Could you check a few things on this model? Use its own coordinates, in mm. A direction names the side the tool comes from. Coordinates: 2 decimals unless noted, no trailing zeros. Loops run counter-clockwise (first coordinate to the right, second up) from the corner with the lowest first, then second, coordinate; pieces in that order, holes last. Notation, with made-up numbers: (52, 80.5) - (62, 80.5) arc R24 ccw to (62, 94.5) - close; hole circle Ø6 at (28, 30.25). An arc over 180 degrees is marked (long way). One line per question, with ' | ' between items. Start each with the question number.
1. I'm going to push flat-ended pins straight in: P1, Ø4, axis at x = -18, y = 7, coming from the -Z side; P2, Ø1.3, axis at x = 77.5, z = -45, coming from the -Y side; P3, Ø0.6, axis at x = -69.5, y = 4.5, coming from the +Z side; P4, Ø0.5, axis at x = -78, y = 1.5, coming from the +Z side. Where does each tip first touch, or does it pass through?
2. I want a section at C-C, the plane z = 25. Write out the boundary of the cut face in (x, y), then the cut area to 3 significant figures.
3. Which directions (+Z, -Z, +X, -X, +Y, -Y) give clear straight access to the entire face, cutting with the end or side of a thin tool? Please do faces 1 (the flat face through (6, 0, 53)), 2 (the flat face through (-73, 5.4, 16)), 3 (the cylindrical face through (-70.64, -0.25, 50.2)).
4. We'd pull the mould along X, two halves only. Please class faces 4 (the cylindrical face through (-78.35, 4.39, 5.28)), 5 (the flat face through (-0.3, 0.5, -43.2)), 6 (the cylindrical face through (70.6, -0.25, -50.24)): pulls with the +X half, pulls with the -X half, needs draft (parallel to the pull), parting line crosses it, or undercut.
5. I want a section at B-B, the plane x = -55.5. Write out the boundary of the cut face in (y, z).
6. Please list where these lines run through material, in increasing order: L1, parallel to X at y = 0.75, z = -44.85; L2, parallel to X at y = 0.75, z = 29; L3, parallel to X at y = 2.25, z = 37. Write a range as [from, to].
7. I want a section at A-A, the plane z = 13.5. Write out the boundary of the cut face in (x, y), then the cut area to 3 significant figures.
from build123d import *

# Parameters (mm, degrees)
SKETCH1_W                            = 159.7
SKETCH1_H                            = 109.7
BOSS_EXTRUDE1_DEPTH                  = 3.4
SKETCH5_W                            = 128
SKETCH5_H                            = 86
CUT_EXTRUDE1_DEPTH                   = 97.933508138
SKETCH6_W                            = 133.6
SKETCH6_H                            = 96.6
CUT_EXTRUDE2_DEPTH                   = 2.9
F_2_7_2_7_DIAMETER_HOLE1_D           = 2.7
F_2_7_2_7_DIAMETER_HOLE1_CSINK_D     = 2.75
F_2_7_2_7_DIAMETER_HOLE1_CSINK_ANGLE = 90
SKETCH10_R                           = 1.35
BOSS_EXTRUDE3_DEPTH                  = 0.5
M2X0_4_TAPPED_HOLE1_D                = 1.6
M2X0_4_TAPPED_HOLE1_CSINK_D          = 2.05
M2X0_4_TAPPED_HOLE1_CSINK_ANGLE      = 90
SKETCH7_W                            = 143
SKETCH7_H                            = 102.2
SKETCH7_W_2                          = 141
SKETCH7_H_2                          = 100.2
BOSS_EXTRUDE2_DEPTH                  = 0.5
SKETCH17_R                           = 1.5
CUT_EXTRUDE6_DEPTH                   = 2
SKETCH15_W                           = 2.5
SKETCH15_H                           = 4.9
CUT_EXTRUDE5_DEPTH                   = 97.952333649
CUT_EXTRUDE4_DEPTH                   = 97.952333649
SKETCH8_R                            = 8
CUT_EXTRUDE3_DEPTH                   = 97.952333649
SKETCH14_R                           = 2.3
BOSS_EXTRUDE4_DEPTH                  = 7.2
FILLET1_R                            = 8
FILLET2_R                            = 2
FILLET3_R                            = 3
FILLET4_R                            = 1
FILLET5_R                            = 2
FILLET6_R                            = 1
SKETCH16_W                           = 13.05
SKETCH16_H                           = 24
BOSS_EXTRUDE5_DEPTH                  = 2
FILLET7_R                            = 5


with BuildPart() as part:
    # Sketch1 → Boss-Extrude1 (new body)
    with BuildSketch(Plane(origin=(0, 0, 0), x_dir=(1, 0, 0), z_dir=(0, 1, 0))):
        Rectangle(SKETCH1_W, SKETCH1_H)
    extrude(amount=BOSS_EXTRUDE1_DEPTH)

    # Sketch5 → Cut-Extrude1 (cut, through all)
    with BuildSketch(Plane.XZ):
        Rectangle(SKETCH5_W, SKETCH5_H)
    extrude(amount=-CUT_EXTRUDE1_DEPTH, mode=Mode.SUBTRACT)

    # Sketch6 → Cut-Extrude2 (cut)
    with BuildSketch(Plane(origin=(0, 3.4, 0), x_dir=(1, 0, 0), z_dir=(0, 1, 0))):
        Rectangle(SKETCH6_W, SKETCH6_H)
    extrude(amount=-CUT_EXTRUDE2_DEPTH, mode=Mode.SUBTRACT)

    # Ø2.7 (2.7) Diameter Hole1 (through all)
    with Locations(Plane(origin=(0, 3.4, 0), x_dir=(1, 0, 0), z_dir=(0, 1, 0))):
        with Locations((-77.5, 29), (-77.5, -29), (77.5, 29), (77.5, -29)):
            CounterSinkHole(F_2_7_2_7_DIAMETER_HOLE1_D / 2, F_2_7_2_7_DIAMETER_HOLE1_CSINK_D / 2, counter_sink_angle=F_2_7_2_7_DIAMETER_HOLE1_CSINK_ANGLE)

    # Sketch10 → Boss-Extrude3 (add)
    with BuildSketch(Plane.XZ):
        with Locations(Location((-77.35, 44.85, 0), (0, 0, 90))):
            Circle(SKETCH10_R)
        with Locations(Location((77.35, -44.85, 0), (0, 0, 90))):
            Circle(SKETCH10_R)
    extrude(amount=BOSS_EXTRUDE3_DEPTH)

    # M2x0.4 Tapped Hole1 (through all)
    with Locations(Plane(origin=(0, -0.5, 0), x_dir=(-1, 0, 0), z_dir=(0, -1, 0))):
        with Locations((-77.35, 44.85), (77.35, -44.85)):
            CounterSinkHole(M2X0_4_TAPPED_HOLE1_D / 2, M2X0_4_TAPPED_HOLE1_CSINK_D / 2, counter_sink_angle=M2X0_4_TAPPED_HOLE1_CSINK_ANGLE)

    # Sketch7 → Boss-Extrude2 (add)
    with BuildSketch(Plane.XZ):
        Rectangle(SKETCH7_W, SKETCH7_H)
        Rectangle(SKETCH7_W_2, SKETCH7_H_2, mode=Mode.SUBTRACT)
    extrude(amount=BOSS_EXTRUDE2_DEPTH)

    # Sketch17 → Cut-Extrude6 (cut)
    with BuildSketch(Plane.XZ):
        with Locations(Location((-76.85, 0, 0), (0, 0, 270))):
            Circle(SKETCH17_R)
        with Locations(Location((76.85, 0, 0), (0, 0, 270))):
            Circle(SKETCH17_R)
    extrude(amount=-CUT_EXTRUDE6_DEPTH, mode=Mode.SUBTRACT)

    # Sketch15 → Cut-Extrude5 (cut, through all)
    with BuildSketch(Plane(origin=(0, 3.4, 0), x_dir=(1, 0, 0), z_dir=(0, 1, 0))):
        with Locations((-78.6, 21.85)):
            Rectangle(SKETCH15_W, SKETCH15_H)
    extrude(amount=-CUT_EXTRUDE5_DEPTH, mode=Mode.SUBTRACT)

    # Sketch9 → Cut-Extrude4 (cut, through all)
    with BuildSketch(Plane(origin=(0, 3.4, 0), x_dir=(1, 0, 0), z_dir=(0, 1, 0))):
        with BuildLine():
            Line((-76.85, 40.85), (-79.85, 40.85))
            Line((-79.85, 40.85), (-79.85, 48.85))
            Line((-79.85, 48.85), (-76.85, 48.85))
            ThreePointArc((-76.85, 48.85), (-72.85, 44.85), (-76.85, 40.85))
        make_face()
    extrude(amount=-CUT_EXTRUDE4_DEPTH, mode=Mode.SUBTRACT)

    # Sketch8 → Cut-Extrude3 (cut, through all)
    with BuildSketch(Plane(origin=(0, 3.4, 0), x_dir=(1, 0, 0), z_dir=(0, 1, 0))):
        with Locations((-79.85, -54.85)):
            Circle(SKETCH8_R)
    extrude(amount=-CUT_EXTRUDE3_DEPTH, mode=Mode.SUBTRACT)

    # Sketch14 → Boss-Extrude4 (add)
    with BuildSketch(Plane(origin=(0, 3.4, 0), x_dir=(1, 0, 0), z_dir=(0, 1, 0))):
        with Locations(Location((-77.35, -44.85, 0), (0, 0, 270))):
            Circle(SKETCH14_R)
        with Locations(Location((77.35, 44.85, 0), (0, 0, 270))):
            Circle(SKETCH14_R)
    extrude(amount=BOSS_EXTRUDE4_DEPTH)

    # Fillet1
    # the kernel refuses this fillet: 8 mm, written as the material it takes off along each edge
    with BuildSketch(Plane(origin=(79.85, -20, 54.85), x_dir=(0, 0, -1), z_dir=(0, 1, 0)), Plane(origin=(79.85, -20, -54.85), x_dir=(-1, 0, 0), z_dir=(0, 1, 0))) as fillet1_piece_1:
        with BuildLine():
            CenterArc((FILLET1_R, FILLET1_R), FILLET1_R, 180, 90)
            Line((0, FILLET1_R), (-FILLET1_R * 0.02, FILLET1_R))
            Line((-FILLET1_R * 0.02, FILLET1_R), (-FILLET1_R * 0.02, -FILLET1_R * 0.02))
            Line((-FILLET1_R * 0.02, -FILLET1_R * 0.02), (FILLET1_R, -FILLET1_R * 0.02))
            Line((FILLET1_R, -FILLET1_R * 0.02), (FILLET1_R, 0))
        make_face()
    extrude(amount=43.4, mode=Mode.SUBTRACT)
    with BuildSketch(Plane(origin=(-79.85, -19.364916731, -54.85), x_dir=(1, 0, 0), z_dir=(0, 1, 0))) as fillet1_piece_2:
        with BuildLine():
            CenterArc((7.745966692, -8), FILLET1_R, 90, 75.522487814)
            Line((0, -6), (-0.154919334, -5.96))
            ThreePointArc((-0.154919334, -5.96), (-0.16, -3), (-0.16, 0))
            Line((-0.16, 0), (0, 0.16))
            Line((0, 0.16), (7.745966692, 0.16))
            Line((7.745966692, 0.16), (7.745966692, 0))
        make_face()
    extrude(amount=42.129833462, mode=Mode.SUBTRACT)

    # Fillet2
    fillet2_edges = [part.edges().sort_by_distance(p)[0] for p in [
        (70.5, -0.25, 50.1),
        (-70.5, -0.25, 50.1),
        (-70.5, -0.25, -50.1),
        (70.5, -0.25, -50.1),
    ]]
    fillet(fillet2_edges, radius=FILLET2_R)

    # Fillet3
    fillet3_edges = [part.edges().sort_by_distance(p)[0] for p in [
        (71.5, -0.25, -51.1),
        (71.5, -0.25, 51.1),
        (-71.5, -0.25, 51.1),
        (-71.5, -0.25, -51.1),
    ]]
    fillet(fillet3_edges, radius=FILLET3_R)

    # Fillet4
    fillet4_edges = [part.edges().sort_by_distance(p)[0] for p in [
        (-64, 0.25, 43),
        (64, 0.25, 43),
        (-64, 0.25, -43),
        (64, 0.25, -43),
    ]]
    fillet(fillet4_edges, radius=FILLET4_R)

    # Fillet5
    fillet5_edges = [part.edges().sort_by_distance(p)[0] for p in [
        (66.8, 1.95, -48.3),
        (66.8, 1.95, 48.3),
        (-66.8, 1.95, 48.3),
        (-66.8, 1.95, -48.3),
    ]]
    fillet(fillet5_edges, radius=FILLET5_R)

    # Fillet6
    fillet6_edges = [part.edges().sort_by_distance(p)[0] for p in [
        (-79.85, 1.7, -19.4),
        (-79.85, 1.7, -24.3),
        (-77.35, 1.7, -24.3),
        (-77.35, 1.7, -19.4),
        (-79.85, 1.7, -40.85),
        (-79.85, 1.7, -48.85),
        (-71.85, 1.7, 54.85),
        (-79.85, 1.7, 46.85),
    ]]
    fillet(fillet6_edges, radius=FILLET6_R)

    # Sketch16 → Boss-Extrude5 (add)
    with BuildSketch(Plane(origin=(0, 3.4, 0), x_dir=(1, 0, 0), z_dir=(0, 1, 0))):
        with Locations((-73.325, -15.85)):
            Rectangle(SKETCH16_W, SKETCH16_H)
    extrude(amount=BOSS_EXTRUDE5_DEPTH)

    # Fillet7
    # the kernel refuses this fillet: 5 mm, written as the material it takes off along each edge
    with BuildSketch(Plane(origin=(-79.85, 3.4, 3.85), x_dir=(0, 0, 1), z_dir=(0, 1, 0))) as fillet7_piece_1:
        with BuildLine():
            CenterArc((FILLET7_R, FILLET7_R), FILLET7_R, 180, 90)
            Line((0, FILLET7_R), (0, 0))
            Line((0, 0), (FILLET7_R, 0))
        make_face()
    extrude(amount=14.5, mode=Mode.SUBTRACT)
    with BuildSketch(Plane(origin=(-79.85, 3.4, 27.85), x_dir=(0, 0, -1), z_dir=(0, 1, 0))) as fillet7_piece_2:
        with BuildLine():
            CenterArc((FILLET7_R, -FILLET7_R), FILLET7_R, 90, 90)
            Line((0, -FILLET7_R), (0, 0))
            Line((0, 0), (FILLET7_R, 0))
        make_face()
    extrude(amount=14.5, mode=Mode.SUBTRACT)


solid = part.part
Results are:
1) P1: passes through | P2: stops at y = -0.34 | P3: stops at z = 27.85 | P4: stops at z = 47.13
2) outline: (-79.85, 0) - (-71.5, 0) - (-71.5, -0.5) - (-70.5, -0.5) - (-70.5, 0) - (-64, 0) - (-64, 0.5) - (-66.8, 0.5) - (-66.8, 5.4) - (-79.36, 5.4) - (-79.36, 3.4) - (-79.85, 3.4) - close; (64, 0) - (70.5, 0) - (70.5, -0.5) - (71.5, -0.5) - (71.5, 0) - (79.85, 0) - (79.85, 3.4) - (66.8, 3.4) - (66.8, 0.5) - (64, 0.5) - close | area: 118 mm2
3) face 1: -Y | face 2: -Z, +X, -X, +Y | face 3: +Z, -X, -Y
4) face 4: pulls with the -X half | face 5: undercut | face 6: pulls with the +X half
5) outline: (-0.5, -51.1) - (0, -51.1) - (0, -54.85) - (3.4, -54.85) - (3.4, -48.3) - (0.5, -48.3) - (0.5, -43) - (0, -43) - (0, -50.1) - (-0.5, -50.1) - close; (-0.5, 50.1) - (0, 50.1) - (0, 43) - (0.5, 43) - (0.5, 48.3) - (3.4, 48.3) - (3.4, 54.85) - (0, 54.85) - (0, 51.1) - (-0.5, 51.1) - close
6) L1: x = [-72.85, -66.8], [66.8, 76.55], [78.15, 79.85] | L2: x = [-79.85, -78.85], [-76.15, -66.8], [66.8, 76.15], [78.85, 79.85] | L3: x = [-79.85, -66.8], [66.8, 79.85]
7) outline: (-79.85, 0) - (-71.5, 0) - (-71.5, -0.5) - (-70.5, -0.5) - (-70.5, 0) - (-64, 0) - (-64, 0.5) - (-66.8, 0.5) - (-66.8, 5.4) - (-79.85, 5.4) - close; (64, 0) - (70.5, 0) - (70.5, -0.5) - (71.5, -0.5) - (71.5, 0) - (79.85, 0) - (79.85, 3.4) - (66.8, 3.4) - (66.8, 0.5) - (64, 0.5) - close | area: 119 mm2
